Geometry check sheet. Reference: the model listing, model coordinates, mm. Coordinates: 2 decimals unless noted, no trailing zeros. Write each loop counter-clockwise with the first axis right and the second up, starting at its lowest first coordinate (ties: lowest second). Pieces come first, ordered by that corner, then holes. Notation, with made-up numbers: (42.5, -23) -> (71.5, -23) arc R34 ccw to (71.5, 10) -> close; hole circle Ø3 at (24, -11). An arc over 180 degrees is marked (long way). One line per question, with ' | ' between items.
```python
from build123d import *

# Parameters (mm, degrees)
SKETCH1_W           = 200
SKETCH1_H           = 240
BOSS_EXTRUDE1_DEPTH = 5
SKETCH3_R           = 8.25
CUT_EXTRUDE1_DEPTH  = 6
SKETCH4_R           = 2.75
CUT_EXTRUDE2_DEPTH  = 6
SKETCH5_R           = 10.75
CUT_EXTRUDE4_DEPTH  = 6
SKETCH6_R           = 3.4
CUT_EXTRUDE5_DEPTH  = 6


with BuildPart() as part:
    # Sketch1 → Boss-Extrude1 (new body)
    with BuildSketch(Plane(origin=(0, 0, 0), x_dir=(1, 0, 0), z_dir=(0, 1, 0))):
        Rectangle(SKETCH1_W, SKETCH1_H)
    extrude(amount=BOSS_EXTRUDE1_DEPTH)

    # Sketch3 → Cut-Extrude1 (cut, through all)
    with BuildSketch(Plane(origin=(0, 5, 0), x_dir=(1, 0, 0), z_dir=(0, 1, 0))):
        with Locations((0, 100)):
            Circle(SKETCH3_R)
    extrude(amount=-CUT_EXTRUDE1_DEPTH, mode=Mode.SUBTRACT)

    # Sketch4 → Cut-Extrude2 (cut, through all)
    with BuildSketch(Plane(origin=(0, 5, 0), x_dir=(1, 0, 0), z_dir=(0, 1, 0))):
        with Locations((19, 100)):
            Circle(SKETCH4_R)
        with Locations((13.435028843, 113.435028843)):
            Circle(SKETCH4_R)
        with Locations((13.435028843, 86.564971157)):
            Circle(SKETCH4_R)
        with Locations((-13.435028843, 86.564971157)):
            Circle(SKETCH4_R)
        with Locations((-19, 100)):
            Circle(SKETCH4_R)
        with Locations((-13.435028843, 113.435028843)):
            Circle(SKETCH4_R)
    extrude(amount=-CUT_EXTRUDE2_DEPTH, mode=Mode.SUBTRACT)

    # Sketch5 → Cut-Extrude4 (cut, through all)
    with BuildSketch(Plane(origin=(0, 5, 0), x_dir=(1, 0, 0), z_dir=(0, 1, 0))):
        with Locations((-60, 100)):
            Circle(SKETCH5_R)
        with Locations((60, 100)):
            Circle(SKETCH5_R)
    extrude(amount=-CUT_EXTRUDE4_DEPTH, mode=Mode.SUBTRACT)

    # Sketch6 → Cut-Extrude5 (cut, through all)
    with BuildSketch(Plane(origin=(0, 5, 0), x_dir=(1, 0, 0), z_dir=(0, 1, 0))):
        with Locations((-48.686291501, 111.313708499)):
            Circle(SKETCH6_R)
        with Locations((-48.686291501, 88.686291501)):
            Circle(SKETCH6_R)
        with Locations((-71.313708499, 88.686291501)):
            Circle(SKETCH6_R)
        with Locations((-71.313708499, 111.313708499)):
            Circle(SKETCH6_R)
    cut_extrude5 = extrude(amount=-CUT_EXTRUDE5_DEPTH, mode=Mode.SUBTRACT)

    # Mirror1: Cut-Extrude5 across plane
    add(cut_extrude5.mirror(Plane(origin=(0, 0, 0), x_dir=(0, 0, 1), z_dir=(1, 0, 0))), mode=Mode.SUBTRACT)


solid = part.part
```
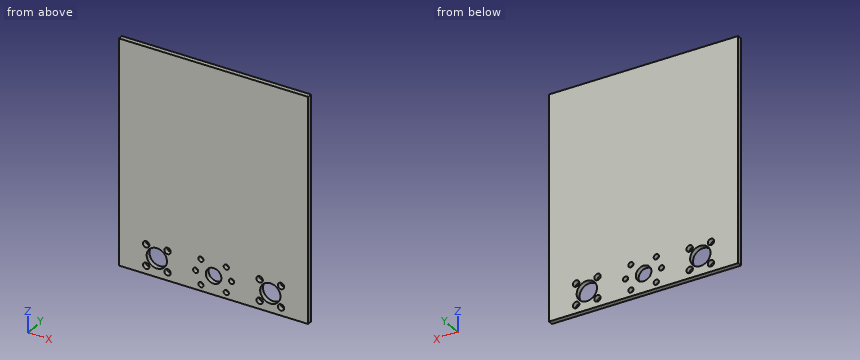
(1) Material ranges on line 1 (X direction, y = 1.65, z = -100); line 2 (Z direction, x = 0, y = 2.25); line 3 (Z direction, x = -71, y = 0.4), recorded low to high.
Answers below:
line 1: x = -100 to -70.75, -49.25 to -21.75, -16.25 to -8.25, 8.25 to 16.25, 21.75 to 49.25, 70.75 to 100 | line 2: z = -120 to -108.25, -91.75 to 120 | line 3: z = -120 to -114.7, -107.93 to -92.07, -85.3 to 120
(2) Cross-section at B-B (z = -100). Record the cut outline in (x, y), plus the area to 4 significant figures.
Answers below:
outline: (-100, 0) -> (-70.75, 0) -> (-70.75, 5) -> (-100, 5) -> close; (-49.25, 0) -> (-21.75, 0) -> (-21.75, 5) -> (-49.25, 5) -> close; (-16.25, 0) -> (-8.25, 0) -> (-8.25, 5) -> (-16.25, 5) -> close; (8.25, 0) -> (16.25, 0) -> (16.25, 5) -> (8.25, 5) -> close; (21.75, 0) -> (49.25, 0) -> (49.25, 5) -> (21.75, 5) -> close; (70.75, 0) -> (100, 0) -> (100, 5) -> (70.75, 5) -> close | area: 647.5 mm²
(3) Cross-section at D-D (x = 19). Record the cut outline in (y, z), plus the area to 3 significant figures.
Answers below:
outline: (0, -120) -> (5, -120) -> (5, -102.75) -> (0, -102.75) -> close; (0, -97.25) -> (5, -97.25) -> (5, 120) -> (0, 120) -> close | area: 1,170 mm²
(4) Cross-section at C-C (y = 4.25). Count the separate pieces of the cut face and the enclosed holes in it, plus the area to 3 significant figures.
Answers below:
separate pieces: 1 | enclosed holes: 17 | area: 46,600 mm²
(5) Cross-section at A-A (x = 60). Record the cut outline in (y, z).
Answers below:
outline: (0, -120) -> (5, -120) -> (5, -110.75) -> (0, -110.75) -> close; (0, -89.25) -> (5, -89.25) -> (5, 120) -> (0, 120) -> close
